Answer from the drawing. Dimensions are ordinates in mm from the lowest x, y and z of the part. A direction names the side the tool comes from. Coordinates: 2 decimals unless noted, no trailing zeros. Write each loop counter-clockwise with the first axis right and the second up, starting at its lowest first coordinate (ties: lowest second). Pieces come first, ordered by that corner, then holes. Notation, with made-up numbers: (38, 76.5) -> (97, 76.5) arc R23 ccw to (97, 87.5) -> close; hole circle Ø3 at (78.5, -35). An arc over 180 degrees is marked (long way). One line per item, written item: value. Start each with the question number.
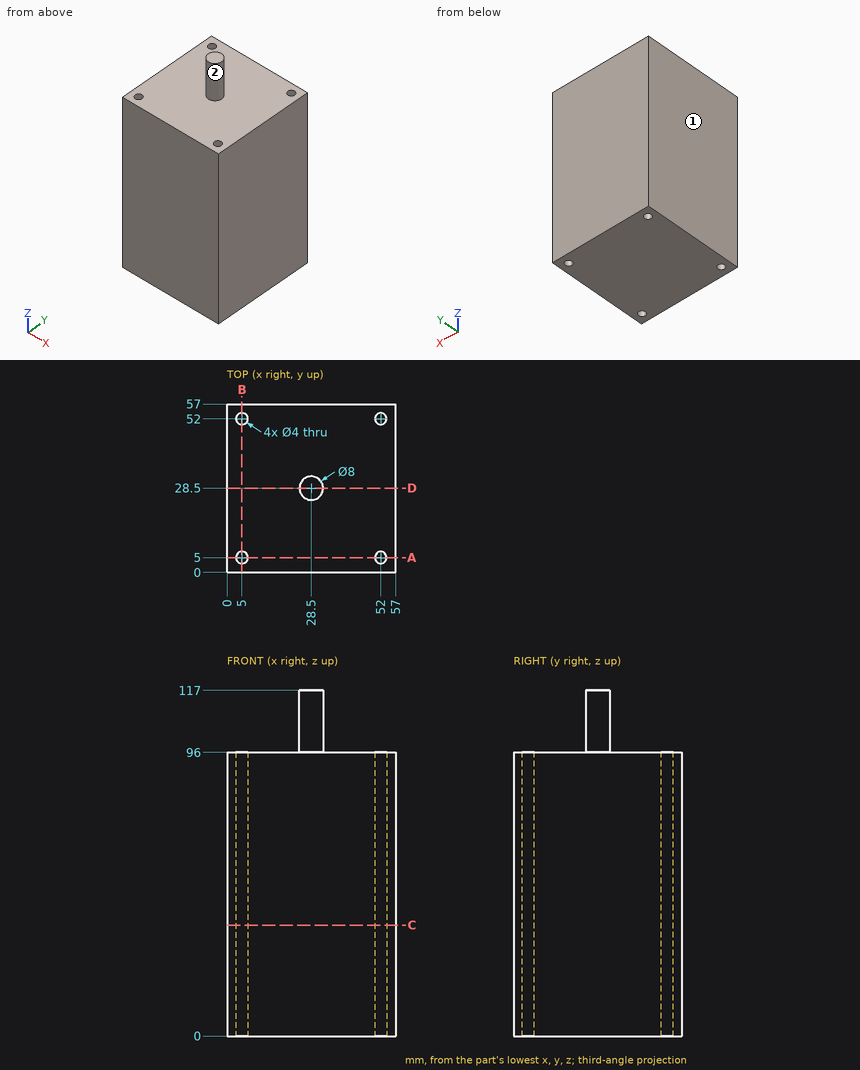
1. Find the intervals of material crossed by probe 1 along Y at (x, z) = (52, 39); probe 2 along Y at (x, z) = (50.5, 7.5), in increasing order. Write a range as from..to.
2. A cutting plane is placed at A-A on y = 5. Give the vertices of the cut face in (x, z).
3. Given pin 1 (3.5 mm diameter, centred on x = 52, y = 52, fed in from -Z), flat-ended and moving along its own axis, determine where the tip first touches the part or whether it passes through.
4. A tool of negligible diameter and unlimited length cuts with its end or side. For the marked faces 1 and 2, from which of +Z, -Z, +X, -X, +Y, -Y can it reach the whole face along a straight path? Write none if from no direction.
5. A cutting plane is placed at C-C on z = 37.5. Give the vertices of the cut face in (x, y).
6. A cutting plane is placed at D-D on y = 28.5. Give the vertices of the cut face in (x, z).
Derived:
1. probe 1: y = 0..3, 7..50, 54..57
1. probe 2: y = 0..3.68, 6.32..50.68, 53.32..57
2. outline: (0, 0) -> (3, 0) -> (3, 96) -> (0, 96) -> close; (7, 0) -> (50, 0) -> (50, 96) -> (7, 96) -> close; (54, 0) -> (57, 0) -> (57, 96) -> (54, 96) -> close
3. pin 1: passes through
4. face 1: +Z, -Z, -X, +Y, -Y
4. face 2: +Z
5. outline: (0, 0) -> (57, 0) -> (57, 57) -> (0, 57) -> close; hole circle Ø4 at (5, 5); hole circle Ø4 at (5, 52); hole circle Ø4 at (52, 5); hole circle Ø4 at (52, 52)
6. outline: (0, 0) -> (57, 0) -> (57, 96) -> (32.5, 96) -> (32.5, 117) -> (24.5, 117) -> (24.5, 96) -> (0, 96) -> close
